```python
from build123d import *

# Parameters (mm, degrees)
F0_W     = 31.75
F0_H     = 15.875
F0_R     = 2.3538427831
F0_R_2   = 2.38125
F1_DEPTH = 3.175
F2_DEPTH = 4.7625
F3_T     = -1.5875
F4_R     = 3.175
F4_R_2   = 2.38125
F5_DEPTH = 1.5875


with BuildPart() as f1:
    # F0 (on Top) → F1 (new body)
    with BuildSketch(Plane.XY):
        with Locations((0, -3.96875)):
            Rectangle(F0_W, F0_H)
        with BuildLine():
            ThreePointArc((-9.5524072169, -7.9375), (-13.5706681938, -9.6019181938), (-11.90625, -5.5836572169))
            ThreePointArc((-11.90625, -5.5836572169), (-10.2418318062, -6.2730818062), (-9.5524072169, -7.9375))
        make_face(mode=Mode.SUBTRACT)
        with Locations((-3.96875, -7.9375)):
            Circle(F0_R, mode=Mode.SUBTRACT)
        with Locations((3.96875, -7.9375)):
            Circle(F0_R, mode=Mode.SUBTRACT)
        with Locations((11.90625, -7.9375)):
            Circle(F0_R, mode=Mode.SUBTRACT)
        with BuildLine():
            ThreePointArc((-11.90625, -2.38125), (-13.5900480227, 1.6837980227), (-9.525, 0))
            ThreePointArc((-9.525, 0), (-10.2224519773, -1.6837980227), (-11.90625, -2.38125))
        make_face(mode=Mode.SUBTRACT)
        with Locations((-3.96875, 0)):
            Circle(F0_R_2, mode=Mode.SUBTRACT)
        with Locations((3.96875, 0)):
            Circle(F0_R_2, mode=Mode.SUBTRACT)
        with Locations((11.90625, 0)):
            Circle(F0_R_2, mode=Mode.SUBTRACT)
    extrude(amount=F1_DEPTH)

    # F0 (on Top) → F2 (join)
    with BuildSketch(Plane.XY):
        with Locations((11.90625, 0)):
            Circle(F0_R_2)
        with BuildLine():
            ThreePointArc((-11.90625, -2.38125), (-10.2224519773, -1.6837980227), (-9.525, 0))
            ThreePointArc((-9.525, 0), (-13.5900480227, 1.6837980227), (-11.90625, -2.38125))
        make_face()
        with Locations((3.96875, 0)):
            Circle(F0_R_2)
        with Locations((-3.96875, 0)):
            Circle(F0_R_2)
        with BuildLine():
            ThreePointArc((-9.5524072169, -7.9375), (-10.2418318062, -6.2730818062), (-11.90625, -5.5836572169))
            ThreePointArc((-11.90625, -5.5836572169), (-13.5706681938, -9.6019181938), (-9.5524072169, -7.9375))
        make_face()
        with Locations((-3.96875, -7.9375)):
            Circle(F0_R)
        with Locations((3.96875, -7.9375)):
            Circle(F0_R)
        with Locations((11.90625, -7.9375)):
            Circle(F0_R)
    extrude(amount=F2_DEPTH)

    # F3
    f3_openings = [f1.faces().sort_by_distance(p)[0] for p in [
        (0, -3.96875, 0),
    ]]
    offset(amount=F3_T, openings=f3_openings, kind=Kind.INTERSECTION)

    # F4 (on face) → F5 (join)
    with BuildSketch(Plane(origin=(0, 0, 1.5875), x_dir=(1, 0, 0), z_dir=(0, 0, -1))):
        with BuildLine():
            Line((-9.6212980227, 5.6525480227), (-10.1825640303, 6.2138140303))
            ThreePointArc((-10.1825640303, 6.2138140303), (-10.1825640303, 1.7236859697), (-5.6924359697, 1.7236859697))
            Line((-5.6924359697, 1.7236859697), (-6.2537019773, 2.2849519773))
            ThreePointArc((-6.2537019773, 2.2849519773), (-9.6212980227, 2.2849519773), (-9.6212980227, 5.6525480227))
        make_face()
        with BuildLine():
            ThreePointArc((-4.7625, 3.96875), (-6.7224801022, 6.9020675157), (-10.1825640303, 6.2138140303))
            Line((-10.1825640303, 6.2138140303), (-9.6212980227, 5.6525480227))
            ThreePointArc((-9.6212980227, 5.6525480227), (-7.0262350767, 6.1687381368), (-5.55625, 3.96875))
            ThreePointArc((-5.55625, 3.96875), (-5.7375118632, 3.0574850767), (-6.2537019773, 2.2849519773))
            Line((-6.2537019773, 2.2849519773), (-5.6924359697, 1.7236859697))
            ThreePointArc((-5.6924359697, 1.7236859697), (-5.0041824843, 2.7537301022), (-4.7625, 3.96875))
        make_face()
        with Locations((0, 3.96875)):
            Circle(F4_R)
        with Locations((0, 3.96875)):
            Circle(F4_R_2, mode=Mode.SUBTRACT)
        with Locations((7.9375, 3.96875)):
            Circle(F4_R)
        with Locations((7.9375, 3.96875)):
            Circle(F4_R_2, mode=Mode.SUBTRACT)
    extrude(amount=F5_DEPTH)


solid = f1.part
```
CAD build for the part. Positions are in the model's coordinates, mm. A direction names the side the tool comes from. Coordinates: 2 decimals unless noted, no trailing zeros. Order: outer loops, then holes, each group sorted by start corner. A loop starts at its lowest first (then second) coordinate and runs counter-clockwise, first axis right, second up. Notation, with made-up numbers: (16, -24) -> (23, -24) arc R15 cw to (23, -1) -> close; hole circle Ø4 at (41.25, 37). An arc over 180 degrees is marked (long way). Use one line per item in the form item = value. Start each with the question number.
1) Band-saw the part on A-A on z = 2.2. State how many separate pieces and enclosed holes the cut face has, then the cut area to 3 significant figures.
2) Band-saw the part on D-D on x = -13. Give the cut face in (y, z) (1 decimal).
3) Tool access for faces 3 (the flat face through (12, -8, 4.762)), 4 (the cylindrical face through (-10.138, -4.879, 0.805)), 5 (the cylindrical face through (6.24, 0.72, 3.96)): list every direction of +Z, -Z, +X, -X, +Y, -Y with a clear straight run to the whole face (end or side of a thin tool).
4) Band-saw the part on C-C on y = 1.75. Give the cut face in (x, z) (1 decimal).
5) Pull direction Y, two halves, no side cores. Call faces 1 (the cylindrical face through (3.36, -8.4, 2.37)), 2 (the flat face through (4, -8, 4.762)): +Y half, -Y half, draft (parallel to the pull), parting line (faces both ways), or undercut.
6) Drill centre lines: L1, parallel to X at y = 0, z = 2.8 (1 decimal); L2, parallel to Y at x = 10, z = 0.6; L3, parallel to Z at x = -6.5, y = -1 (1 decimal). Where is each one in solid material? Low to high. Write a range as [from, to].
7) Drop flat-ended pins along their axis: pin 1 (1.2 mm diameter, centred on x = 4, y = -8, fed in from -Z) (3 decimals); pin 2 (1.8 mm diameter, centred on x = -11.91, y = 0, fed in from -Z). Give the stop position or say it passes through.
Entries:
q1.separate_pieces = 1
q1.enclosed_holes = 8
q1.area = 489 mm2
q2.outline = (-11.9, 0) -> (-10.3, 0) -> (-10.3, 1.6) -> (2.4, 1.6) -> (2.4, 0) -> (4, 0) -> (4, 3.2) -> (2.1, 3.2) -> (2.1, 4.8) -> (-2.1, 4.8) -> (-2.1, 3.2) -> (-5.9, 3.2) -> (-5.9, 4.8) -> (-10, 4.8) -> (-10, 3.2) -> (-11.9, 3.2) -> close
q3.face_3 = +Z, +X, -X, +Y, -Y
q3.face_4 = -Z
q3.face_5 = +Z
q4.outline = (-15.9, 0) -> (-14.3, 0) -> (-14.3, 1.6) -> (14.3, 1.6) -> (14.3, 0) -> (15.9, 0) -> (15.9, 3.2) -> (13.5, 3.2) -> (13.5, 4.8) -> (10.3, 4.8) -> (10.3, 3.2) -> (5.6, 3.2) -> (5.6, 4.8) -> (2.4, 4.8) -> (2.4, 3.2) -> (-2.4, 3.2) -> (-2.4, 4.8) -> (-5.6, 4.8) -> (-5.6, 3.2) -> (-10.3, 3.2) -> (-10.3, 4.8) -> (-13.5, 4.8) -> (-13.5, 3.2) -> (-15.9, 3.2) -> close
q5.face_1 = undercut
q5.face_2 = draft
q6.L1 = [-15.9, -12.7], [-11.1, -4.8], [-3.2, 3.2], [4.8, 11.1], [12.7, 15.9]
q6.L2 = [-11.91, -10.32], [-6.38, -5.16], [-2.78, -1.55], [2.38, 3.97]
q6.L3 = [1.6, 3.2]
q7.pin_1 = 3.175
q7.pin_2 = 1.59
